Build history of the part. All positions in model axes, mm. Give positions to 0.01 mm unless a question says otherwise; leave off trailing zeros. Loops run counter-clockwise (first coordinate to the right, second up) from the corner with the lowest first, then second, coordinate; pieces in that order, holes last. Notation, with made-up numbers: (43, 33.5) -> (56, 33.5) arc R33 cw to (56, 67.5) -> close; hole circle Ø3 at (-38.5, 52). An arc over 180 degrees is marked (long way). One line per question, with ' | ' between items. Start each with the question number.
(1) Drill centre lines: L1, parallel to Z at x = 17.25, y = 6.35; L2, parallel to Y at x = -22, z = -11.75; L3, parallel to X at y = 5.75, z = 1. Where is each one in solid material? Low to high. Write a range as from..to.
(2) Flat gauge pin, fed straight in: pin 1 Ø1.6 at (y, z) = (6.35, -0.02) entering from -X. Where does the tip first touch, or does it go through?
(3) Slice it at A-A, the plane x = -14.5. Write the cut outline in (y, z).
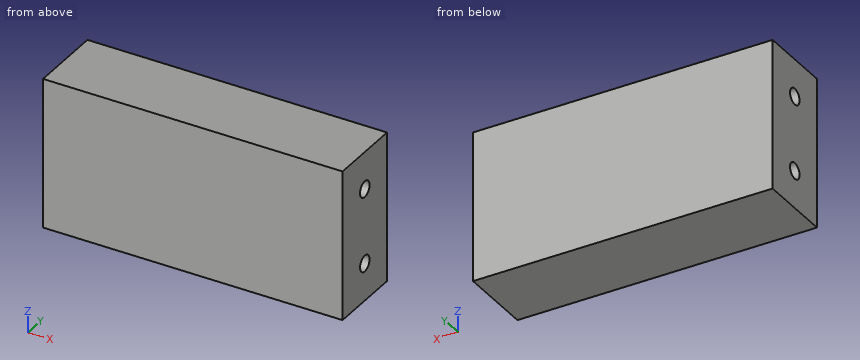
```python
from build123d import *

# Parameters (mm, degrees)
SKETCH1_W                      = 50.8
SKETCH1_H                      = 25.4
BOSS_EXTRUDE1_DEPTH            = 12.7
F_6_32_TAPPED_HOLE1_AT_2_COUNT = 2
F_6_32_TAPPED_HOLE1_AT_2_PITCH = 12.7


with BuildPart() as part:
    # Sketch1 → Boss-Extrude1 (new body)
    with BuildSketch(Plane(origin=(0, 0, 0), x_dir=(1, 0, 0), z_dir=(0, 1, 0))):
        with Locations((-0.6, 6.366666667)):
            Rectangle(SKETCH1_W, SKETCH1_H)
    extrude(amount=BOSS_EXTRUDE1_DEPTH)

    # Sketch3 → #6-32 Tapped Hole1 (revolve, cut)
    with BuildSketch(Plane(origin=(24.8, 6.35, -0.016666667), x_dir=(0, 0, -1), z_dir=(0, 1, 0))):
        Polygon((0, 0), (0, 13.51269403), (1.35255, 12.7), (1.35255, 0), align=None)
    f_6_32_tapped_hole1 = revolve(axis=Axis((31.15, 6.35, -0.016666667), (-1, 0, 0)), mode=Mode.SUBTRACT)

    # #6-32 Tapped Hole1 at 2: #6-32 Tapped Hole1 ×2
    with Locations(*[(0, 0, -i * F_6_32_TAPPED_HOLE1_AT_2_PITCH) for i in range(1, F_6_32_TAPPED_HOLE1_AT_2_COUNT)]):
        add(f_6_32_tapped_hole1, mode=Mode.SUBTRACT)

    # Mirror1: #6-32 Tapped Hole1 across plane
    add(f_6_32_tapped_hole1.mirror(Plane(origin=(-0.6, 0, 0), x_dir=(0, 0, 1), z_dir=(1, 0, 0))), mode=Mode.SUBTRACT)

    # Mirror1 copy 1 sketch → Mirror1 copy 1 (revolve, cut)
    with BuildSketch(Plane(origin=(-26, 6.35, -12.716666667), x_dir=(0, 0, -1), z_dir=(0, 1, 0))):
        Polygon((0, 0), (0, -13.51269403), (1.35255, -12.7), (1.35255, 0), align=None)
    revolve(axis=Axis((-32.35, 6.35, -12.716666667), (-1, 0, 0)), mode=Mode.SUBTRACT)


solid = part.part
```
Final values:
1) L1: -19.07..-14.07, -11.36..-1.37, 1.34..6.33 | L2: 0..5.4, 7.3..12.7 | L3: -13.2..12
2) pin 1: x = -12.97
3) outline: (0, -19.07) -> (12.7, -19.07) -> (12.7, 6.33) -> (0, 6.33) -> close; hole circle Ø2.71 at (6.35, -12.72); hole circle Ø2.71 at (6.35, -0.02)
